```python
from build123d import *

# Parameters (mm, degrees)
ODEBRAT_VYSUNUT_M1_DEPTH = 5
ODEBRAT_VYSUNUT_M2_DEPTH = 8
KRUHOV_POLE1_COUNT       = 12


with BuildPart() as part:
    # Skica1 → Rotovat1 (revolve)
    with BuildSketch(Plane(origin=(0, 0, 0), x_dir=(0, 0, -1), z_dir=(1, 0, 0))):
        Polygon((2.75, 0), (8, 0), (10, 2), (10, 5), (8, 7), (2.75, 7), align=None)
    revolve(axis=Axis((0, 0, 0), (0, 1, 0)))

    # Skica2 → Odebrat vysunutím1 (cut)
    with BuildSketch(Plane(origin=(0, 7, 0), x_dir=(1, 0, 0), z_dir=(0, 1, 0))):
        Polygon((-4, -2.309401077), (0, -4.618802154), (4, -2.309401077), (4, 2.309401077), (0, 4.618802154), (-4, 2.309401077), align=None)
    extrude(amount=-ODEBRAT_VYSUNUT_M1_DEPTH, mode=Mode.SUBTRACT)

    # Skica3 → Odebrat vysunutím2 (cut, through all)
    with BuildSketch(Plane(origin=(0, 7, 0), x_dir=(1, 0, 0), z_dir=(0, 1, 0))):
        with BuildLine():
            Line((-1, 8.94427191), (-1.5, 9.886859967))
            ThreePointArc((-1.5, 9.886859967), (0, 10), (1.5, 9.886859967))
            Line((1.5, 9.886859967), (1, 8.94427191))
            ThreePointArc((1, 8.94427191), (0, 9), (-1, 8.94427191))
        make_face()
    odebrat_vysunut_m2 = extrude(amount=-ODEBRAT_VYSUNUT_M2_DEPTH, mode=Mode.SUBTRACT)

    # Kruhové pole1: Odebrat vysunutím2 ×12 about axis
    kruhov_pole1_axis = Axis((0, 0, 0), (0, 1, 0))
    for i in range(1, KRUHOV_POLE1_COUNT):
        add(odebrat_vysunut_m2.rotate(kruhov_pole1_axis, i * 360 / KRUHOV_POLE1_COUNT), mode=Mode.SUBTRACT)


solid = part.part
```
Work out the finished part from the listing and answer in its coordinate system (mm). A direction names the side the tool comes from. Give positions to 0.01 mm unless a question says otherwise; leave off trailing zeros. Order: outer loops, then holes, each group sorted by start corner. A loop starts at its lowest first (then second) coordinate and runs counter-clockwise, first axis right, second up. Notation, with made-up numbers: M 19,-35.75 L 46,-35.75 A12 ccw 46,-19.75 Z; hole C 13.5,17 d4. An arc over 180 degrees is marked long. Return JSON: item names as keys, results as strings.
1) For a pull along Z with two mould halves and no side action, classify faces 4 (the flat face through (9.422, 3.535, 1.254)), 5 (the cylindrical face through (2.573, 3.521, 9.663)), 6 (the cylindrical face through (2.603, 3.521, -9.655)) as +Z half, -Z half, draft (parallel to the pull), parting line (faces both ways), or undercut.
Resolved:
{"face 4": "undercut", "face 5": "+Z half", "face 6": "-Z half"}
2) Straight lines are drawn through the part: line 1 along Z through (x, y) = (0, 1.4); line 2 along Z through (x, y) = (7.5, 3.5); line 3 along X through (y, z) = (3, 7.75). For each, find the intervals that lie inside material, in ascending order. Write a range as [from, to].
Resolved:
{"line 1": "[-9, -2.75], [2.75, 9]", "line 2": "[-6.61, -5.74], [-4.97, 4.97], [5.74, 6.61]", "line 3": "[-6.32, -6.14], [-4.58, 4.58], [6.14, 6.32]"}
3) A tool of negligible diameter and unlimited length cuts with its end or side. For faces 1 (the flat face through (7.533, 3.535, 5.797)), 2 (the flat face through (-7.533, 3.535, -5.797)), 3 (the flat face through (-1.254, 3.535, 9.422)), from which of +Z, -Z, +X, -X, +Y, -Y can it reach the whole face along a straight path? Write none if from no direction.
Resolved:
{"face 1": "+X, +Y, -Y", "face 2": "-X, +Y, -Y", "face 3": "+Z, +Y, -Y"}
4) Each of these flat-tipped pins is pushed along its axis until it touches: pin 1 (5 mm diameter, centred on x = 0, z = 0, fed in from -Y); pin 2 (9 mm diameter, centred on x = 0, z = -1, fed in from +Y); pin 3 (1.5 mm diameter, centred on y = 1.5, z = 6.5, fed in from +X). Where does it stop, or does it pass through?
Resolved:
{"pin 1": "through", "pin 2": "y = 7", "pin 3": "x = 7.81"}
5) Section B-B, the plane z = 0 is taken. Write down the section's boundary in (x, y), plus the area to 3 significant figures.
Resolved:
{"outline": "M -9,1 L -8,0 L -2.75,0 L -2.75,2 L -4,2 L -4,7 L -8,7 L -9,6 Z; M 2.75,0 L 8,0 L 9,1 L 9,6 L 8,7 L 4,7 L 4,2 L 2.75,2 Z", "area": "73.0 mm^2"}
6) Section A-A, the plane y = 6.25 is taken. Write down the section's boundary in (x, z).
Resolved:
{"outline": "C 0,0 d17.5; hole M -4,-2.31 L 0,-4.62 L 4,-2.31 L 4,2.31 L 0,4.62 L -4,2.31 Z"}
